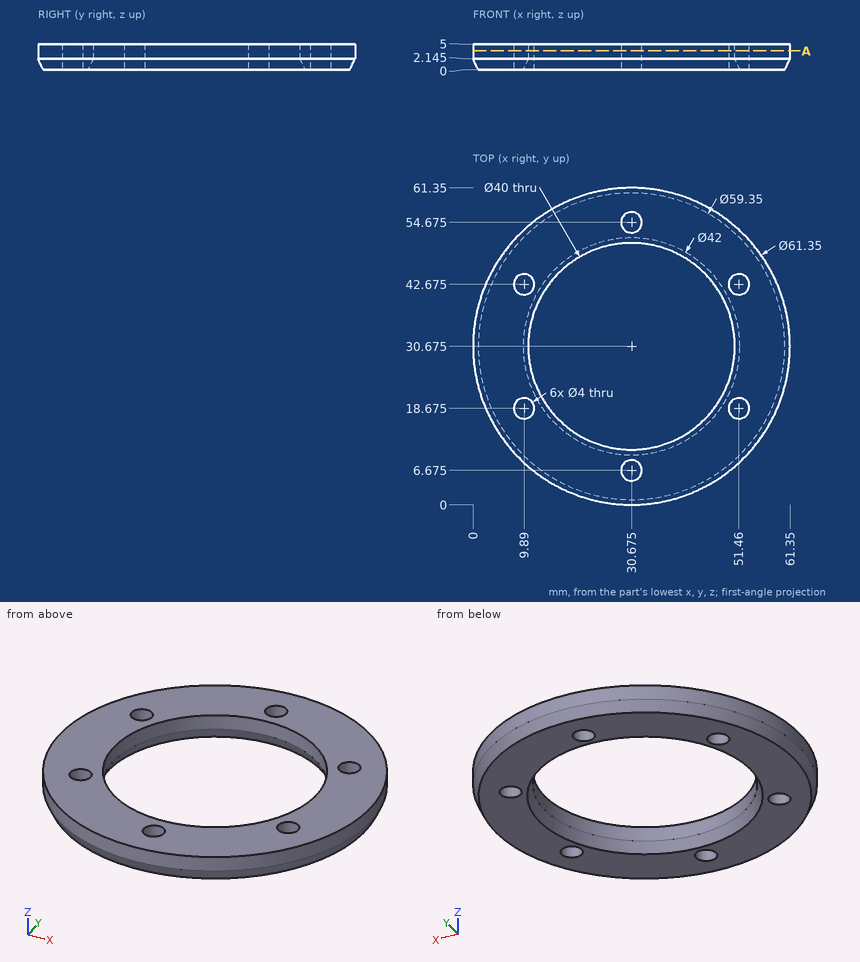
Study the drawing (mm; zero at the part's minimum x, y, z) and answer. Round coordinates to 2 decimals unless told otherwise and drop trailing zeros. One line per item, written item: value.
Q1. Flat-ended cylindrical pins translate along their axes: pin 1 (24 mm diameter, centred on x = 30.675, y = 30.675, fed in from -Z); pin 2 (1.5 mm diameter, centred on y = 12, z = 4.5, fed in from +X); pin 3 (2 mm diameter, centred on y = 11.5, z = 4, fed in from -X) (1 decimal); pin 4 (1.5 mm diameter, centred on y = 49.5, z = 2.5, fed in from -X). Find the tip coordinate at first contact, or state that the pin passes through.
Derived:
pin 1: through
pin 2: x = 55.57
pin 3: x = 6
pin 4: x = 5.89
Q2. Straight lines are drawn through the part: line 1 (Y direction, x = 8.5, z = 3.35) (1 decimal); line 2 (Y direction, x = 10, z = 3.8) (1 decimal); line 3 (X direction, y = 20.5, z = 2.45) (1 decimal). For each, find the intervals that lie inside material, in ascending order.
Derived:
line 1: 9.5 to 17.2, 20.1 to 41.2, 44.1 to 51.9
line 2: 8 to 16.7, 20.7 to 40.7, 44.7 to 53.3
line 3: 1.7 to 9.1, 10.7 to 13.5, 47.9 to 50.6, 52.3 to 59.6
Q3. Find section A-A on z = 3.65. Give the number of separate pieces and of enclosed holes in the cut face, then the cut area to 3 significant figures.
Derived:
separate pieces: 1
enclosed holes: 7
area: 1,620 mm²
